Verification items for the finished model (mm, model axes). Coordinates: 2 decimals unless noted, no trailing zeros. Order: outer loops, then holes, each group sorted by start corner. A loop starts at its lowest first (then second) coordinate and runs counter-clockwise, first axis right, second up. Notation, with made-up numbers: M 18,89 L 24,89 A14 cw 24,111 Z; hole C 29,15 d1. An arc over 180 degrees is marked long. Answer as a JSON object with one key per item and string values. Group by question number.
(1) Gauge pin test, flat ends, axial feed: pin 1 Ø4 at (y, z) = (102, 26.5) entering from -X; pin 2 Ø1.5 at (y, z) = (80, 136.5) entering from +X; pin 3 Ø12 at (y, z) = (97, 46.5) entering from -X. Record the tip position at first contact, or that the pin passes through.
(2) Cross-section at B-B (y = 48). Enter the section's corners in (x, z).
(3) Cross-section at A-A (x = -48). Enter the section's corners in (y, z).
(4) Material ranges on line 1 (X direction, y = 105, z = 58); line 2 (X direction, y = 56, z = 136.5); line 3 (Y direction, x = -31, z = 122), recorded low to high.
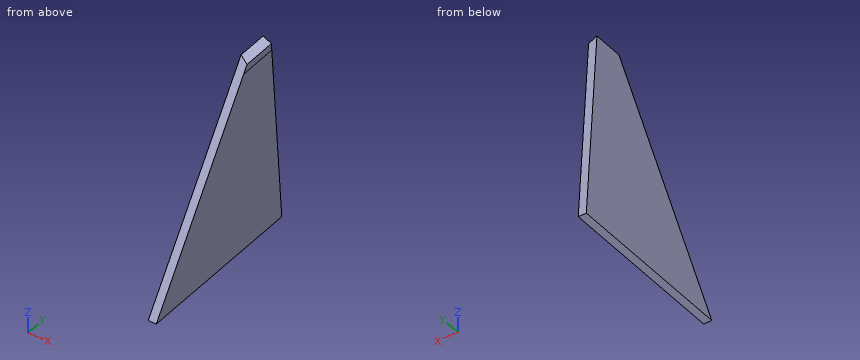
from build123d import *

# Parameters (mm, degrees)
BOSS_EXTRUDE1_DEPTH = 152.4
SKETCH3_OUTSIDE_W   = 273.93
SKETCH3_OUTSIDE_H   = 229.576
CUT_EXTRUDE2_DEPTH  = 381.660734008
SHELL1_T            = -6.35
CUT_EXTRUDE3_DEPTH  = 381.660734008
CUT_EXTRUDE4_DEPTH  = 332.131034202


with BuildPart() as part:
    # Sketch2 → Boss-Extrude1 (new body)
    with BuildSketch(Plane(origin=(0, 0, 0), x_dir=(1, 0, 0), z_dir=(0, 1, 0))):
        Polygon((-57.15, 0), (224.536, 0), (-24.357683353, -196.753899884), align=None)
    extrude(amount=BOSS_EXTRUDE1_DEPTH)

    # Sketch3 outside → Cut-Extrude2 (cut, through all)
    with BuildSketch(Plane(origin=(-63.5, 0, 0), x_dir=(0, 0, -1), z_dir=(1, 0, 0))):
        with Locations((-98.377, 76.2)):
            Rectangle(SKETCH3_OUTSIDE_W, SKETCH3_OUTSIDE_H)
        Polygon((0, 152.4), (-152.4, 107.95), (-261.257142857, 76.2), (-152.4, 44.45), (0, 0), align=None, mode=Mode.SUBTRACT)
    extrude(amount=CUT_EXTRUDE2_DEPTH, mode=Mode.SUBTRACT)

    # Shell1
    shell1_openings = [part.faces().sort_by_distance(p)[0] for p in [
        (83.693, 76.2, 0),
    ]]
    offset(amount=SHELL1_T, openings=shell1_openings, kind=Kind.INTERSECTION)

    # Sketch4 → Cut-Extrude3 (cut, through all)
    with BuildSketch(Plane(origin=(-63.5, 0, 0), x_dir=(0, 0, -1), z_dir=(1, 0, 0))):
        Polygon((0, 152.4), (0, 145.785416667), (-196.753899884, 88.398862534), (-196.753899884, 95.013445867), align=None)
        Polygon((-196.753899884, 64.001137466), (0, 6.614583333), (0, 0), (-196.753899884, 57.386554133), align=None)
    extrude(amount=CUT_EXTRUDE3_DEPTH, mode=Mode.SUBTRACT)

    # Sketch5 → Cut-Extrude4 (cut, through all)
    with BuildSketch(Plane(origin=(0, 149.86, 0), x_dir=(1, 0, 0), z_dir=(0, 1, 0))):
        Polygon((-19.861548271, -185.105168304), (-18.669521453, -192.257329212), (344.317071882, -192.257329212), (317.879717865, 72.864270331), (-35.136715197, 43.31663937), align=None)
    extrude(amount=-CUT_EXTRUDE4_DEPTH, mode=Mode.SUBTRACT)


solid = part.part
Taken from the geometry:
{
 "1": {"pin 1": "stops at x = -53.07", "pin 2": "stops at x = -27.84", "pin 3": "stops at x = -50.4"},
 "2": {"outline": "M -57.15,0 L -50.71,0 L -27.06,141.89 L -33.5,141.89 Z"},
 "3": {"outline": "M 11.36,16.27 L 141.04,16.27 L 129.77,54.9 L 22.63,54.9 Z"},
 "4": {"line 1": "x = -47.48 to -41.05", "line 2": "x = -34.4 to -27.96", "line 3": "y = 42.2 to 110.2"}
}
